Part print with two shaded views. Sizes in mm from the minimum x, y, z corner. Give positions to 0.01 mm unless a question says otherwise; leave off trailing zeros. Write each loop counter-clockwise with the first axis right and the second up, starting at its lowest first coordinate (ties: lowest second). Pieces come first, ordered by that corner, then holes. Notation, with made-up numbers: (65.5, 70.5) -> (107.5, 70.5) arc R17 cw to (107.5, 74.5) -> close; hole circle Ø7 at (-15.75, -2.5). An arc over 180 degrees is marked (long way). Answer as a JSON object with one key per item and string values.
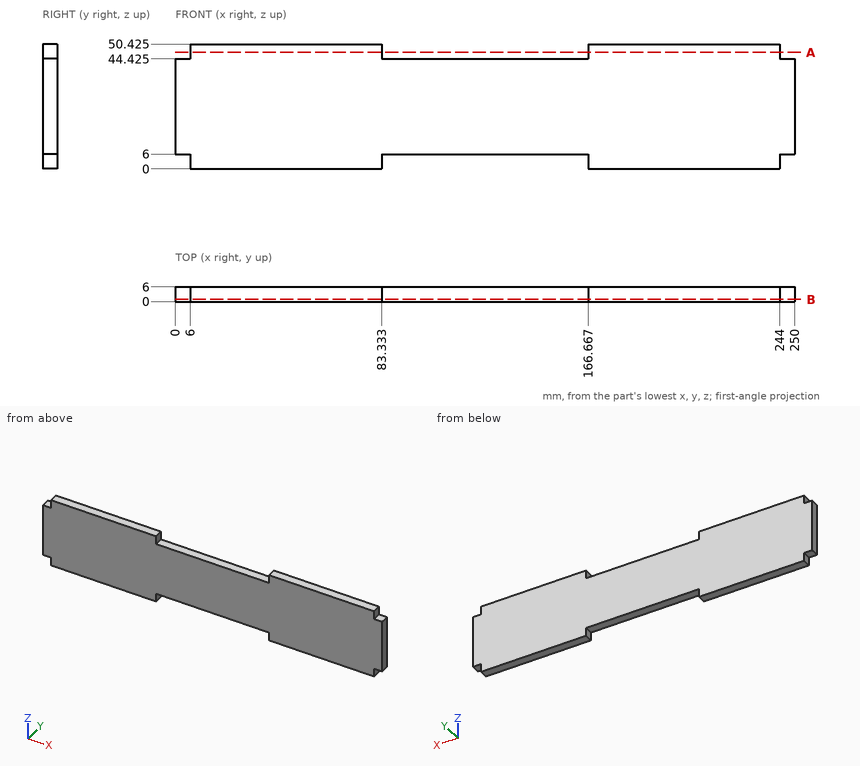
1) Wall check: probe 1 along X at (y, z) = (4.6, 46.5); probe 2 along Z at (x, y) = (116, 4.45) (1 decimal). Give the ranges that are in metal, low to high.
Model answer:
{"probe 1": "x = 6 to 83.33, 166.67 to 244", "probe 2": "z = 6 to 44.4"}
2) Slice it at B-B (y = 1). List the corners of the cut face in (x, z) (1 decimal).
Model answer:
{"outline": "(0, 6) -> (6, 6) -> (6, 0) -> (83.3, 0) -> (83.3, 6) -> (166.7, 6) -> (166.7, 0) -> (244, 0) -> (244, 6) -> (250, 6) -> (250, 44.4) -> (244, 44.4) -> (244, 50.4) -> (166.7, 50.4) -> (166.7, 44.4) -> (83.3, 44.4) -> (83.3, 50.4) -> (6, 50.4) -> (6, 44.4) -> (0, 44.4) -> close"}
3) Pin check, flat tips, straight feed: pin 1 (1.8 mm diameter, centred on y = 2, z = 47.5, fed in from -X); pin 2 (3 mm diameter, centred on x = 133.5, y = 4, fed in from -Z); pin 3 (1.8 mm diameter, centred on y = 4, z = 2.5, fed in from +X). Stop position of each tip, or through.
Model answer:
{"pin 1": "stops at x = 6", "pin 2": "stops at z = 6", "pin 3": "stops at x = 244"}
4) Slice it at A-A (z = 47). List the corners of the cut face in (x, y), then the cut area to 3 significant figures.
Model answer:
{"outline": "(6, 0) -> (83.33, 0) -> (83.33, 6) -> (6, 6) -> close; (166.67, 0) -> (244, 0) -> (244, 6) -> (166.67, 6) -> close", "area": "928 mm2"}
